from build123d import *

# Parameters (mm, degrees)
SKETCH1_R           = 10
SKETCH1_R_2         = 9
BOSS_EXTRUDE1_DEPTH = 10
CUT_EXTRUDE1_REACH  = 19.321


with BuildPart() as part:
    # Sketch1 → Boss-Extrude1 (new body)
    with BuildSketch(Plane(origin=(0, 0, 0), x_dir=(1, 0, 0), z_dir=(0, 1, 0))):
        with Locations(Location((0, 0, 0), (0, 0, 270))):
            Circle(SKETCH1_R)
        with Locations(Location((0, 0, 0), (0, 0, 270))):
            Circle(SKETCH1_R_2, mode=Mode.SUBTRACT)
    extrude(amount=BOSS_EXTRUDE1_DEPTH)

    # Sketch3 → Cut-Extrude1 (cut, up to next)
    with BuildSketch(Plane.XY, mode=Mode.PRIVATE) as cut_extrude1_sk1:
        Polygon((0, 0), (-5.773502692, 10), (-5.42709253, 10), (0.346410162, 0), align=None)
    cut_extrude1_tool1 = extrude(cut_extrude1_sk1.sketch, amount=-CUT_EXTRUDE1_REACH, mode=Mode.PRIVATE) & part.part
    add(cut_extrude1_tool1.solids().sort_by_distance((-2.713546, 5, 0))[0], mode=Mode.SUBTRACT)


solid = part.part
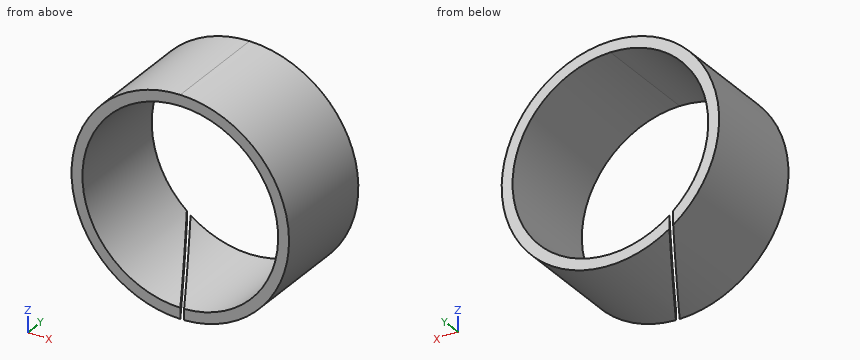
Can you work these out from the model? Positions are in its coordinate system, mm. Give positions to 0.01 mm unless a question says otherwise; leave off trailing zeros. Order: outer loops, then holes, each group sorted by start corner. A loop starts at its lowest first (then second) coordinate and runs counter-clockwise, first axis right, second up. Notation, with made-up numbers: M 66,86 L 100,86 A9 cw 100,93 Z; hole C 4,-21.75 d2. An arc over 180 degrees is marked long. Use one line per item in the form item = value.
Item 1: Will these pins go through, and if not, where does the flat tip stop? pin 1 Ø2 at (x, y) = (5.5, 3) entering from -Z; pin 2 Ø1.5 at (y, z) = (2, -2.5) entering from +X; pin 3 Ø5 at (y, z) = (8, -3.5) entering from -X.
Values follow:
pin_1 = -8.93
pin_2 = 9.85
pin_3 = -9.95
Item 2: If we section it at B-B, the plane x = -4: Write out the boundary of the cut face in (y, z).
Values follow:
outline = M 0,-9.17 L 6.93,-9.17 L 6.93,-8.06 L 0,-8.06 Z; M 0,8.06 L 10,8.06 L 10,9.17 L 0,9.17 Z; M 7.53,-9.17 L 10,-9.17 L 10,-8.06 L 7.53,-8.06 Z
Item 3: If I drill on line 1 along Z through (x, y) = (0, 7.25); line 2 along X through (y, z) = (7.75, 2), over which ranges is the centre line in solid material (lowest first)? Write a range as [from, to].
Values follow:
line_1 = [-10, -9], [9, 10]
line_2 = [-9.8, -8.77], [8.77, 9.8]
Item 4: If we section it at A-A, the plane z = 0: Write out the boundary of the cut face in (x, y).
Values follow:
outline = M -10,0 L -9,0 L -9,10 L -10,10 Z; M 9,0 L 10,0 L 10,10 L 9,10 Z
Item 5: If we section it at C-C, the plane z = 5.5: Write out the boundary of the cut face in (x, y), and give its area (3 significant figures).
Values follow:
outline = M -8.35,0 L -7.12,0 L -7.12,10 L -8.35,10 Z; M 7.12,0 L 8.35,0 L 8.35,10 L 7.12,10 Z
area = 24.6 mm^2
Item 6: If we section it at D-D, the plane y = 5.25: Write out the boundary of the cut face in (x, z).
Values follow:
outline = M -3.03,-9.53 L -3.03,-8.47 A9 cw long -2.68,-8.59 L -2.68,-9.63 A10 ccw long Z
